The listing builds one solid part. Answer for the finished solid, in the listing's coordinates (mm). Give positions to 0.01 mm unless a question says otherwise; leave off trailing zeros. Write each loop counter-clockwise with the first axis right and the second up, starting at its lowest first coordinate (ties: lowest second). Pieces come first, ordered by that corner, then holes. Notation, with made-up numbers: M 31,14.25 L 72,14.25 A10 cw 72,22.25 Z; hole C 62,-3.75 d7. An arc over 180 degrees is marked long. Return JSON: item names as keys, results as strings.
from build123d import *

# Parameters (mm, degrees)
F0_W           = 56.849372
F0_H           = 50.102681
F1_DEPTH       = 25
F3_D           = 5
F3_CSINK_D     = 10
F3_CSINK_ANGLE = 90
F5_D           = 5
F5_CSINK_D     = 10
F5_CSINK_ANGLE = 90
F6_D           = 5
F6_CBORE_D     = 10
F6_CBORE_DEPTH = 5


with BuildPart() as f1:
    # F0 (on Front) → F1 (new body)
    with BuildSketch(Plane.XZ):
        with Locations((72.599741, -7.349261)):
            Rectangle(F0_W, F0_H)
    extrude(amount=F1_DEPTH)

    # F3 (through all)
    with Locations(Plane.XZ.offset(25)):
        with Locations((72.959617, 0)):
            CounterSinkHole(F3_D / 2, F3_CSINK_D / 2, counter_sink_angle=F3_CSINK_ANGLE)

    # F5 (through all)
    with Locations(Plane.YZ.offset(101.024427)):
        with Locations((-13.537139, 0)):
            CounterSinkHole(F5_D / 2, F5_CSINK_D / 2, counter_sink_angle=F5_CSINK_ANGLE)

    # F6 (through all)
    with Locations(Plane.YZ.offset(101.024427)):
        with Locations((-13.537139, 0)):
            CounterBoreHole(F6_D / 2, F6_CBORE_D / 2, F6_CBORE_DEPTH)


solid = f1.part
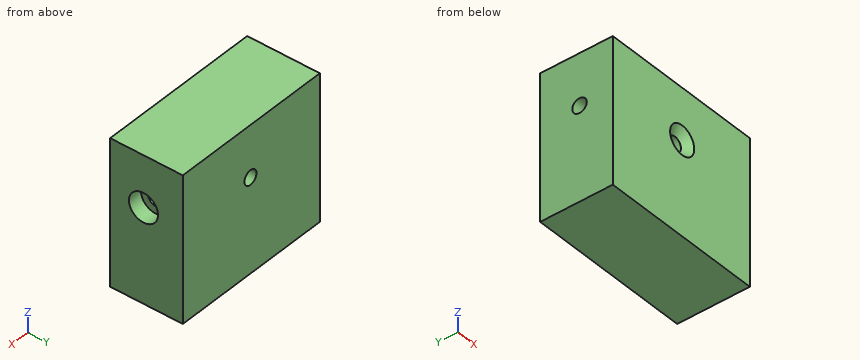
Item 1: A cutting plane is placed at B-B, the plane x = 88.5. Write down the section's boundary in (y, z), plus the area to 3 significant figures.
Geometry results:
{"outline": "M -25,-32.4 L 0,-32.4 L 0,17.7 L -25,17.7 Z; hole C -13.54,0 d5", "area": "1,230 mm2"}
Item 2: A cutting plane is placed at A-A, the plane z = 0. Write down the section's boundary in (x, y).
Geometry results:
{"outline": "M 44.18,-25 L 67.96,-25 L 70.46,-22.5 L 70.46,-16.04 L 44.18,-16.04 Z; M 44.18,-11.04 L 70.46,-11.04 L 70.46,0 L 44.18,0 Z; M 75.46,-22.5 L 77.96,-25 L 101.02,-25 L 101.02,-18.54 L 96.02,-18.54 L 96.02,-16.04 L 75.46,-16.04 Z; M 75.46,-11.04 L 96.02,-11.04 L 96.02,-8.54 L 101.02,-8.54 L 101.02,0 L 75.46,0 Z"}
Item 3: A cutting plane is placed at C-C, the plane y = -10. Write down the section's boundary in (x, z), plus the area to 3 significant figures.
Geometry results:
{"outline": "M 44.18,-32.4 L 101.02,-32.4 L 101.02,-3.53 L 96.02,-3.53 L 96.02,3.53 L 101.02,3.53 L 101.02,17.7 L 44.18,17.7 Z; hole C 72.96,0 d5", "area": "2,790 mm2"}
Item 4: Given pin 1 Ø8 at (x, z) = (72.96, 0) entering from -Y; pin 2 Ø6 at (y, z) = (-13.54, 0) entering from +X; pin 3 Ø6 at (x, z) = (72.96, 0) entering from -Y; pin 4 Ø4.5 at (y, z) = (-13.54, 0) entering from +X, each flat-ended and moving along its own axis, determine where each tip first touches the part or whether it passes through.
Geometry results:
{"pin 1": "stops at y = -24", "pin 2": "stops at x = 96.02", "pin 3": "stops at y = -23", "pin 4": "passes through"}
Item 5: Find the intervals of material crossed by line 1 (X direction, y = -19, z = 0); line 2 (Y direction, x = 56.25, z = 0); line 3 (Y direction, x = 97, z = 0), in increasing order.
Geometry results:
{"line 1": "x = 44.18 to 70.46, 75.46 to 101.02", "line 2": "y = -25 to -16.04, -11.04 to 0", "line 3": "y = -25 to -18.54, -8.54 to 0"}
